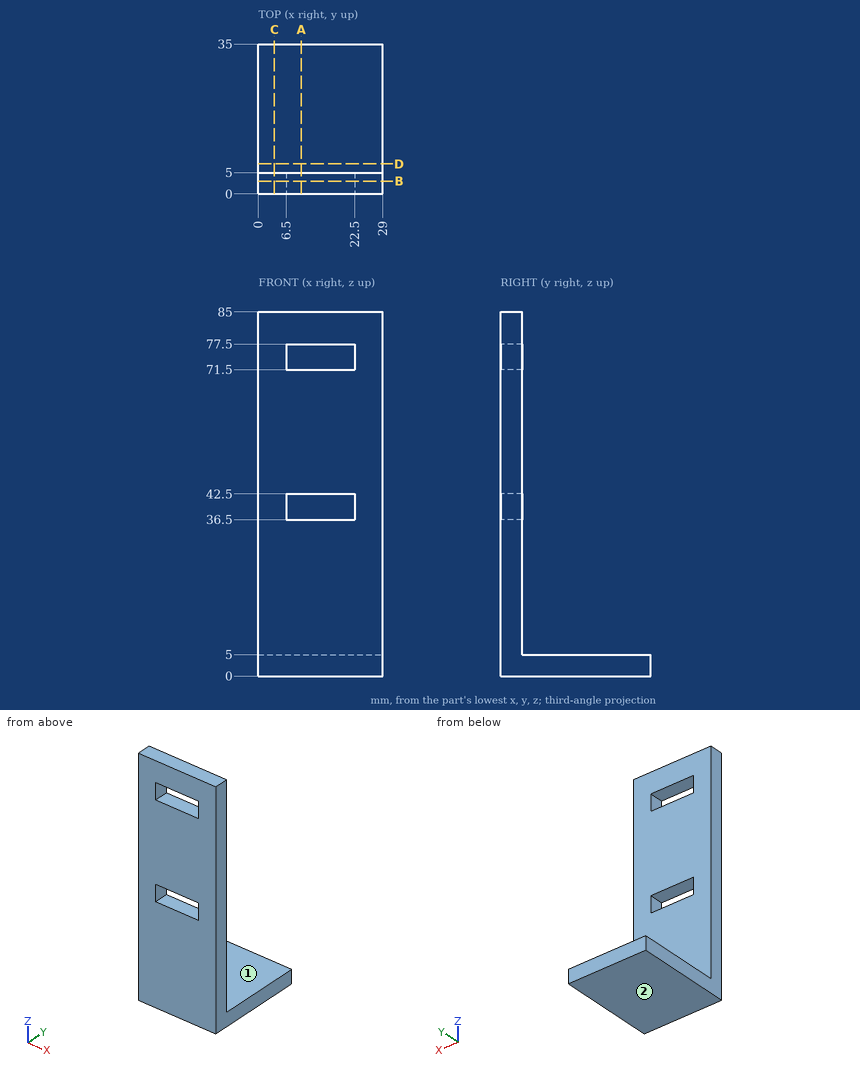
The figure shows three views and two pictorial views of one solid part (mm, origin at its lowest corner). Answer the questions. A direction names the side the tool comes from. Round coordinates to 2 decimals unless told otherwise and drop trailing zeros. Order: outer loops, then holes, each group sorted by start corner. A loop starts at its lowest first (then second) coordinate and runs counter-clockwise, first axis right, second up. Notation, with made-up numbers: M 16.5,86.25 L 43.5,86.25 A36 cw 43.5,125.25 Z; hole C 78.25,58 d6. An arc over 180 degrees is marked long. Put each result on its own line as item: value. Start each with the question number.
Q1. Section D-D, the plane y = 7 is taken. Write down the section's boundary in (x, z).
Q2. A tool of negligible diameter and unlimited length cuts with its end or side. For the marked faces 1 and 2, from which of +Z, -Z, +X, -X, +Y, -Y can it reach the whole face along a straight path? Write none if from no direction.
Q3. Section B-B, the plane y = 3 is taken. Write down the section's boundary in (x, z).
Q4. Section C-C, the plane x = 3.75 is taken. Write down the section's boundary in (y, z).
Q5. Section A-A, the plane x = 10 is taken. Write down the section's boundary in (y, z), and give its area (3 significant figures).
Q6. A straight line is drawn through the part: L1, parallel to Y at x = 26, z = 81. Find the intervals that lie inside material, in ascending order. Write a range as [from, to].
Q7. Flat-ended cylindrical pins translate along their axes: pin 1 (8 mm diameter, centred on x = 7.5, z = 32.5, fed in from +Y); pin 2 (6 mm diameter, centred on y = 8.5, z = 28, fed in from +X) (3 decimals); pin 3 (14.5 mm diameter, centred on x = 8, y = 18, fed in from +Z). Find the tip coordinate at first contact, or state that the pin passes through.
Findings below:
1. outline: M 0,0 L 29,0 L 29,5 L 0,5 Z
2. face 1: +Z, +X, -X, +Y
2. face 2: -Z, +X, -X, +Y, -Y
3. outline: M 0,0 L 29,0 L 29,85 L 0,85 Z; hole M 6.5,36.5 L 22.5,36.5 L 22.5,42.5 L 6.5,42.5 Z; hole M 6.5,71.5 L 22.5,71.5 L 22.5,77.5 L 6.5,77.5 Z
4. outline: M 0,0 L 35,0 L 35,5 L 5,5 L 5,85 L 0,85 Z
5. outline: M 0,0 L 35,0 L 35,5 L 5,5 L 5,36.5 L 0,36.5 Z; M 0,42.5 L 5,42.5 L 5,71.5 L 0,71.5 Z; M 0,77.5 L 5,77.5 L 5,85 L 0,85 Z
5. area: 515 mm^2
6. L1: y = [0, 5]
7. pin 1: stops at y = 5
7. pin 2: passes through
7. pin 3: stops at z = 5
